CAD build for the part. Positions are in the model's coordinates, mm. Give positions to 0.01 mm unless a question says otherwise; leave off trailing zeros. Write each loop counter-clockwise with the first axis right and the second up, starting at its lowest first coordinate (ties: lowest second). Pieces come first, ordered by that corner, then holes. Notation, with made-up numbers: (-31.75, 38.5) - (-14.75, 38.5) arc R25 cw to (-14.75, 71.5) - close; hole circle Ø11 at (-38, 48.25). An arc over 180 degrees is marked (long way). Answer as a JSON object with one key per item and string values.
from build123d import *

# Parameters (mm, degrees)
SKETCH_W        = 76.2
SKETCH_H        = 76.2
PAD_DEPTH       = 5
SKETCH001_R     = 25.4
POCKET_DEPTH    = 5.001
SKETCH002_R     = 2.25
POCKET001_DEPTH = 5.001


with BuildPart() as part:
    # Sketch → Pad (new body)
    with BuildSketch(Plane.XY):
        Rectangle(SKETCH_W, SKETCH_H)
    extrude(amount=PAD_DEPTH)

    # Sketch001 (on Face6 of Pad) → Pocket (cut, through all)
    with BuildSketch(Plane.XY.offset(5)):
        Circle(SKETCH001_R)
    extrude(amount=-POCKET_DEPTH, mode=Mode.SUBTRACT)

    # Sketch002 (on Face5 of Pocket) → Pocket001 (cut, through all)
    with BuildSketch(Plane.XY.offset(5)):
        with Locations((-30.1, -30.1)):
            Circle(SKETCH002_R)
        with Locations((30.1, -30.1)):
            Circle(SKETCH002_R)
        with Locations((30.1, 30.1)):
            Circle(SKETCH002_R)
        with Locations((-30.1, 30.1)):
            Circle(SKETCH002_R)
    extrude(amount=-POCKET001_DEPTH, mode=Mode.SUBTRACT)


solid = part.part
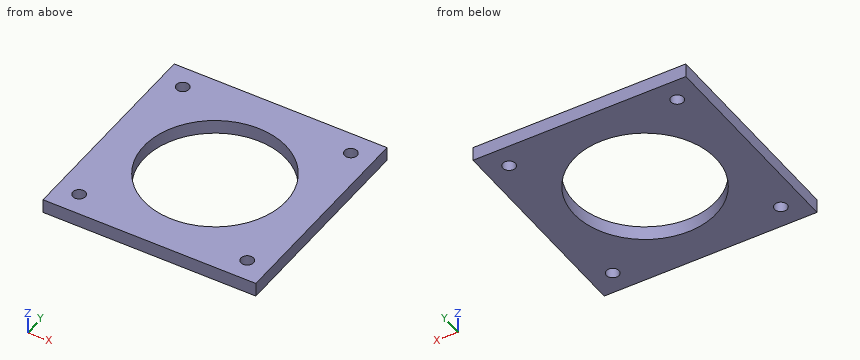
Item 1: Flat gauge pin, fed straight in: P1, Ø7, axis at x = -30.1, y = 30.1, coming from the -Z side. Where does the tip first touch, or does it go through?
Entries:
{"P1": "z = 0"}
Item 2: Probe line 1 (Y direction, x = 30.1, z = 4); line 2 (X direction, y = -30.5, z = 2.5); line 3 (Y direction, x = -28.5, z = 2.3). List the from-to ranges inside material, lowest first. Write a range as from..to.
Entries:
{"line 1": "-38.1..-32.35, -27.85..27.85, 32.35..38.1", "line 2": "-38.1..-32.31, -27.89..27.89, 32.31..38.1", "line 3": "-38.1..-31.68, -28.52..28.52, 31.68..38.1"}
Item 3: Cut at A-A (y = -30.1). Give the cut face in (x, z).
Entries:
{"outline": "(-38.1, 0) - (-32.35, 0) - (-32.35, 5) - (-38.1, 5) - close; (-27.85, 0) - (27.85, 0) - (27.85, 5) - (-27.85, 5) - close; (32.35, 0) - (38.1, 0) - (38.1, 5) - (32.35, 5) - close"}
Item 4: Cut at C-C (y = 0). Give the cut face in (x, z), and give its area (3 significant figures).
Entries:
{"outline": "(-38.1, 0) - (-25.4, 0) - (-25.4, 5) - (-38.1, 5) - close; (25.4, 0) - (38.1, 0) - (38.1, 5) - (25.4, 5) - close", "area": "127 mm2"}
